from build123d import *

# Parameters (mm, degrees)
SKICA1_R                 = 2
P_IDAT_VYSUNUT_M3_DEPTH  = 2
ODEBRAT_START            = -18
SKICA5_R                 = 2.5
SKICA5_R_2               = 2
ODEBRAT_VYSUNUT_M1_DEPTH = 18


with BuildPart() as part:
    # Skica1 → Přidat vysunutím3 (new body)
    # profile 1 of 2: a face of its own
    with BuildSketch(Plane(origin=(0, 0, 0), x_dir=(1, 0, 0), z_dir=(0, 1, 0))):
        with BuildLine():
            Line((108.040914438, 105.971068272), (106.006427981, 34.226677149))
            ThreePointArc((106.006427981, 34.226677149), (110.004588085, 37.999997369), (113.994081517, 34.217515135))
            Line((113.994081517, 34.217515135), (112.040914438, 106))
            Line((112.040914438, 106), (110, 111.642221926))
            Line((110, 111.642221926), (108.040914438, 105.971068272))
        make_face()
    # profile 2 of 2: a face of its own
    with BuildSketch(Plane(origin=(0, 0, 0), x_dir=(1, 0, 0), z_dir=(0, 1, 0))):
        with BuildLine():
            ThreePointArc((106, 34), (107.171572875, 31.171572875), (110, 30))
            ThreePointArc((110, 30), (112.828427125, 31.171572875), (114, 34))
            Line((114, 34), (113.994081517, 34.217515135))
            ThreePointArc((113.994081517, 34.217515135), (110.004588085, 37.999997369), (106.006427981, 34.226677149))
            Line((106.006427981, 34.226677149), (106, 34))
        make_face()
        with Locations(Location((110, 34, 0), (0, 0, 270))):
            Circle(SKICA1_R, mode=Mode.SUBTRACT)
    extrude(amount=P_IDAT_VYSUNUT_M3_DEPTH)

    # Skica5 → Odebrat vysunutím1 (cut)
    with BuildSketch(Plane(origin=(0, 2, 0), x_dir=(1, 0, 0), z_dir=(0, 1, 0)).offset(ODEBRAT_START)):
        with Locations(Location((110, 34, 0), (0, 0, 270))):
            Circle(SKICA5_R)
        with Locations((110, 34)):
            Circle(SKICA5_R_2, mode=Mode.SUBTRACT)
    extrude(amount=ODEBRAT_VYSUNUT_M1_DEPTH, mode=Mode.SUBTRACT)


solid = part.part
Verification items for the finished model (mm, model axes). Coordinates: 2 decimals unless noted, no trailing zeros. Order: outer loops, then holes, each group sorted by start corner. A loop starts at its lowest first (then second) coordinate and runs counter-clockwise, first axis right, second up. Notation, with made-up numbers: (21, 30) -> (48, 30) arc R35 cw to (48, 68) -> close; hole circle Ø7 at (71.25, 59). An arc over 180 degrees is marked (long way). Put each result on its own line as item: value. Start each with the question number.
1. Material ranges on L1, parallel to X at y = 0.7, z = -34; L2, parallel to X at y = 0.55, z = -90.5; L3, parallel to X at y = 1, z = -51, recorded low to high. Write a range as [from, to].
2. Cross-section at C-C, the plane z = -107. Record the boundary of the cut face in (x, y).
3. Go/stop test with flat-tipped pins: pin 1 Ø1 at (x, z) = (111.5, -57) entering from -Y; pin 2 Ø1 at (x, y) = (111, 1) entering from +Z; pin 3 Ø1 at (y, z) = (1, -55.5) entering from -X. Record where each tip stops, or that it passes through.
4. Cross-section at A-A, the plane y = 1.65. Record the boundary of the cut face in (x, z), then the cut area to 3 significant figures.
5. Mould release check, pull along Z, two halves, no side actions. Record for faces 1 (the flat face through (110, 2, -71)), 2 (the flat face through (109.034, 0.986, -108.846)), 3 (the cylindrical face through (112.48, 0.99, -34.33)): released by +Z, released by -Z, zero draft, split by the parting line, or undercut.
6. Cross-section at B-B, the plane z = -93. Record the boundary of the cut face in (x, y).
Computed:
1. L1: [106, 107.5], [112.5, 114]
1. L2: [107.6, 112.46]
1. L3: [106.48, 113.54]
2. outline: (108.4, 0) -> (111.68, 0) -> (111.68, 2) -> (108.4, 2) -> close
3. pin 1: y = 0
3. pin 2: z = -30.03
3. pin 3: x = 106.6
4. outline: (106, -34) -> (108.04, -105.97) -> (110, -111.64) -> (112.04, -106) -> (114, -34) arc R4 ccw to start; hole circle Ø5 at (110, -34)
4. area: 449 mm2
5. face 1: zero draft
5. face 2: released by -Z
5. face 3: undercut
6. outline: (107.67, 0) -> (112.39, 0) -> (112.39, 2) -> (107.67, 2) -> close
